from build123d import *

# Parameters (mm, degrees)
BOSS_EXTRUDE1_REACH      = 44.981
BOSS_EXTRUDE1_END_RADIUS = 15
BOSS_EXTRUDE1_START      = -17
SKETCH2_R                = 10
CHAMFER1_SIZE            = 1


with BuildPart() as part:
    # Sketch1 → Revolve1 (revolve)
    with BuildSketch(Plane.XY):
        with BuildLine():
            Line((11.842719282, 4), (14.456832295, 4))
            ThreePointArc((14.456832295, 4), (11.937336386, -9.082951062), (0, -15))
            Line((0, -15), (0, -12.5))
            ThreePointArc((0, -12.5), (10.155048006, -7.288689869), (11.842719282, 4))
        make_face()
    revolve(axis=Axis((0, 23.994682016, 0), (0, -1, 0)))

    # Boss-Extrude1: up to this sphere (the profile starts outside it)
    boss_extrude1_end = Location((0, 0, 0)) * Sphere(BOSS_EXTRUDE1_END_RADIUS, mode=Mode.PRIVATE)
    # Sketch2 → Boss-Extrude1 (add, up to the surface)
    with BuildSketch(Plane(origin=(0, 0, 0), x_dir=(1, 0, 0), z_dir=(0, 1, 0)).offset(BOSS_EXTRUDE1_START), mode=Mode.PRIVATE) as boss_extrude1_sk1:
        with Locations(Location((0, 0, 0), (0, 0, 180))):
            Circle(SKETCH2_R)
    boss_extrude1_tool1 = extrude(boss_extrude1_sk1.sketch, amount=BOSS_EXTRUDE1_REACH, mode=Mode.PRIVATE) - boss_extrude1_end
    add(boss_extrude1_tool1.solids().sort_by_distance((0, -17, 0))[0])

    # Chamfer1
    # the kernel refuses this chamfer: 1, 0.789005964 mm, written as the material it takes off along each edge
    with BuildSketch(Plane(origin=(0, 4, 0), x_dir=(1, 0, 0), z_dir=(0, 0, -1))) as chamfer1_piece_1:
        with BuildLine():
            Line((11.842719282 + CHAMFER1_SIZE, 0), (12.074893395, 0.767825887))
            ThreePointArc((12.074893395, 0.767825887), (11.967702274, 0.391107888), (11.842719282, 0))
            Line((11.842719282, 0), (11.842719282 + CHAMFER1_SIZE, 0))
        make_face()
    revolve(axis=Axis((0, 4, 0), (0, -1, 0)), mode=Mode.SUBTRACT)


solid = part.part
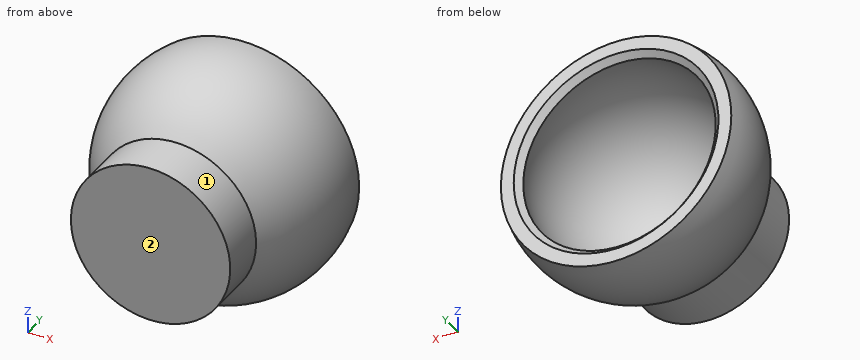
Geometry: final body of the model. Coordinates: model frame, mm. Face numbers are marked on the shaded views. A direction names the side the tool comes from. Give positions to 0.01 mm unless a question says otherwise; leave off trailing zeros. Loops run counter-clockwise (first coordinate to the right, second up) from the corner with the lowest first, then second, coordinate; pieces in that order, holes last. Notation, with made-up numbers: (58.25, 22) -> (112.25, 22) arc R22 cw to (112.25, 32) -> close; hole circle Ø6 at (-7, 44.25). An arc over 180 degrees is marked (long way). Put each result on its own line as item: value.
1. Cut plane D-D (y = -13). Return the cut outline in (x, z).
Taken from the geometry:
outline: circle Ø20 at (0, 0)
2. Pin query (flat end, axial travel): P1, Ø6, axis at y = -3, z = -3, coming from the -X side; P2, Ø3, axis at y = -12, z = -9, coming from the +X side; P3, Ø1.5, axis at x = -8.5, y = -9, coming from the +Z side. Return the tip coordinate at first contact, or that it passes through.
Taken from the geometry:
P1: stops at x = -14.95
P2: stops at x = 6.61
P3: stops at z = 9.47
3. Set-up query: the marked faces 1 and 2. Return all of +Z, -Z, +X, -X, +Y, -Y with unobstructed straight access to the full face (end or side cutting, diameter ignored); none if empty.
Taken from the geometry:
face 1: -Y
face 2: +Z, -Z, +X, -X, -Y
4. Ray query, line 1 along Y through (x, z) = (-1, -5.5); line 2 along Z through (x, y) = (-4, 2.5); line 3 along X through (y, z) = (1, 9). Return the intervals inside material, ascending. Write a range as [from, to].
Taken from the geometry:
line 1: y = [-17, -11.18]
line 2: z = [-14.24, -11.58], [11.58, 14.24]
line 3: x = [-11.96, -8.62], [8.62, 11.96]
5. Cut plane A-A (x = 0). Return the cut outline in (y, z), plus the area to 3 significant figures.
Taken from the geometry:
outline: (-17, -10) -> (-11.18, -10) arc R15 ccw to (4, -14.46) -> (4, -12.84) -> (3.23, -12.07) arc R12.5 cw (long way) to (3.23, 12.07) -> (4, 12.84) -> (4, 14.46) arc R15 ccw to (-11.18, 10) -> (-17, 10) -> close
area: 192 mm2
6. Cut plane C-C (z = 0). Return the cut outline in (x, y), plus the area to 3 significant figures.
Taken from the geometry:
outline: (-14.46, 4) arc R15 ccw to (-10, -11.18) -> (-10, -17) -> (10, -17) -> (10, -11.18) arc R15 ccw to (14.46, 4) -> (12.84, 4) -> (12.07, 3.23) arc R12.5 cw (long way) to (-12.07, 3.23) -> (-12.84, 4) -> close
area: 192 mm2
7. Cut plane B-B (y = -2). Return the cut outline in (x, z).
Taken from the geometry:
outline: circle Ø29.73 at (0, 0); hole circle Ø24.68 at (0, 0)
